Geometry: see drawing. Coordinates: mm, zero at the bounding-box minimum. A direction names the side the tool comes from. Give positions to 0.01 mm unless a question says otherwise; leave off trailing zeros. Loops run counter-clockwise (first coordinate to the right, second up) from the corner with the lowest first, then second, coordinate; pieces in that order, holes last. Notation, with made-up numbers: (-28, 70.5) -> (-9, 70.5) arc R10 cw to (-9, 79.5) -> close; hole circle Ø3 at (-28, 29.5). An arc over 180 degrees is marked (long way). Use CSV: the item, a comma, the result in double quotes.
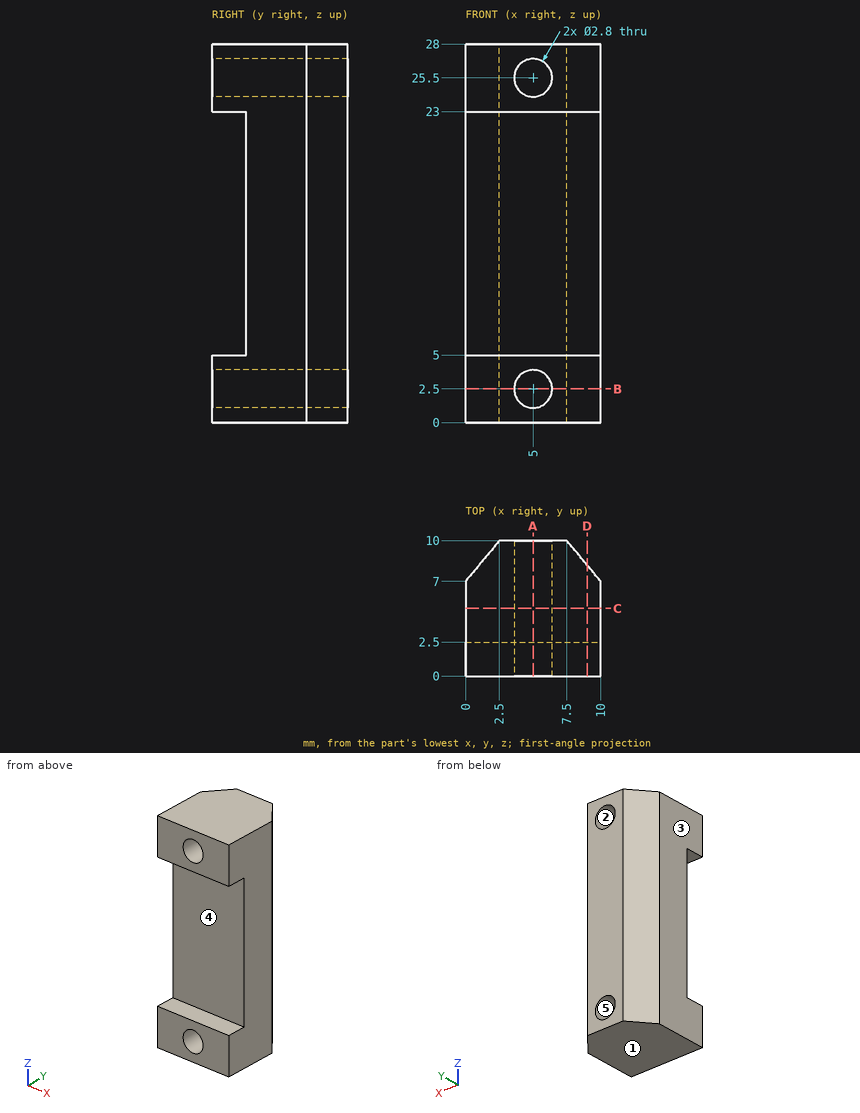
1) Section query C-C (y = 5). Return loops of the section in (x, z).
From the geometry:
outline,"(0, 0) -> (10, 0) -> (10, 28) -> (0, 28) -> close; hole circle Ø2.8 at (5, 2.5); hole circle Ø2.8 at (5, 25.5)"
2) Section query D-D (x = 9). Return loops of the section in (y, z).
From the geometry:
outline,"(0, 0) -> (8.2, 0) -> (8.2, 28) -> (0, 28) -> (0, 23) -> (2.5, 23) -> (2.5, 5) -> (0, 5) -> close"
3) Section query A-A (x = 5). Return loops of the section in (y, z).
From the geometry:
outline,"(0, 0) -> (10, 0) -> (10, 1.1) -> (0, 1.1) -> close; (0, 3.9) -> (10, 3.9) -> (10, 24.1) -> (0, 24.1) -> (0, 23) -> (2.5, 23) -> (2.5, 5) -> (0, 5) -> close; (0, 26.9) -> (10, 26.9) -> (10, 28) -> (0, 28) -> close"
4) Ray query, line 1 (Z direction, x = 5, y = 3.5); line 2 (Z direction, x = 4.5, y = 6.5); line 3 (Y direction, x = 3.5, z = 10). Return the intervals inside material, ascending.
From the geometry:
line 1,"z = 0 to 1.1, 3.9 to 24.1, 26.9 to 28"
line 2,"z = 0 to 1.19, 3.81 to 24.19, 26.81 to 28"
line 3,"y = 2.5 to 10"
5) Mould query, pull axis X, two halves, no side actions, for the marked faces 1, 2 and 3. Classes: pulls with the +X half, pulls with the -X half, needs draft (parallel to the pull), parting line crosses it, or undercut.
From the geometry:
face 1,"needs draft"
face 2,"undercut"
face 3,"pulls with the -X half"
6) Section query B-B (z = 2.5). Return loops of the section in (x, y), then the cut area to 3 significant figures.
From the geometry:
outline,"(0, 0) -> (3.6, 0) -> (3.6, 10) -> (2.5, 10) -> (0, 7) -> close; (6.4, 0) -> (10, 0) -> (10, 7) -> (7.5, 10) -> (6.4, 10) -> close"
area,"64.5 mm^2"
7) Reachability of the marked faces 4 and 5 from +Z, -Z, +X, -X, +Y, -Y: full face, straight path, thin tool, end or side. Return the list, or none.
From the geometry:
face 4,"+X, -X, -Y"
face 5,"+Y, -Y"
8) Contact query for flat-ended pins moving along their axis: pin 1 (2.5 mm diameter, centred on x = 5, z = 25.5, fed in from +Y) (1 decimal); pin 2 (2 mm diameter, centred on x = 2, z = 7, fed in from -Y). Output: stop coordinate, or through.
From the geometry:
pin 1,"passes through"
pin 2,"stops at y = 2.5"
